Check sheet for the modelled part. Datum: model origin and axes. Units: mm. Round coordinates to 2 decimals unless told otherwise and drop trailing zeros. Order: outer loops, then holes, each group sorted by start corner. A loop starts at its lowest first (then second) coordinate and runs counter-clockwise, first axis right, second up. Notation, with made-up numbers: M 73,74 L 112,74 A23 ccw 112,82 Z; hole C 72,55.25 d7. An arc over 180 degrees is marked long. One line per item, written item: value. Start each with the question number.
(1) Cross-section at C-C, the plane y = 1.75. Enter the section's corners in (x, z).
(2) Cross-section at A-A, the plane x = -20. Enter the section's corners in (y, z).
(3) Cross-section at B-B, the plane z = 0.95. Enter the section's corners in (x, y).
(4) Release check for a two-part mould opening along X. For faces 1 (the face through (-20.737, 16.705, 0.986)), 2 (the face through (-22.5, 8, 1)), 3 (the face through (-17.5, 9, 1)), 4 (the face through (-20, 9, 2)) record: released by +X, released by -X, zero draft, split by the parting line, or undercut.
(5) Thickness scan on L1, parallel to Y at x = -20, z = 1.5; L2, parallel to X at y = 16, z = 0.9; L3, parallel to X at y = 0.5, z = 1.25. Record the ranges inside material, lowest first.
(6) Depth check by flat-ended pin: pin 1 Ø1.6 at (x, y) = (-20, 1.03) entering from -Z; pin 2 Ø2.5 at (x, y) = (-20, 16.03) entering from -Z. Enter the tip coordinate at first touch or a pass-through.
from build123d import *

# Parameters (mm, degrees)
SKETCH_1_R      = 1
EXTRUDE_2_DEPTH = 2
FILLET_1_R      = 0.3


with BuildPart() as part:
    # 草图1 → 凸台-拉伸2 (new body)
    with BuildSketch(Plane.XY):
        with BuildLine():
            Line((-22.5, 1.029411765), (-22.5, 16.029411765))
            ThreePointArc((-22.5, 16.029411765), (-20, 18.529411765), (-17.5, 16.029411765))
            Line((-17.5, 16.029411765), (-17.5, 1.029411765))
            ThreePointArc((-17.5, 1.029411765), (-20, -1.470588235), (-22.5, 1.029411765))
        make_face()
        with Locations((-20, 16.029411765)):
            Circle(SKETCH_1_R, mode=Mode.SUBTRACT)
        with Locations((-20, 1.029411765)):
            Circle(SKETCH_1_R, mode=Mode.SUBTRACT)
    extrude(amount=EXTRUDE_2_DEPTH)

    # 圆角1
    fillet_1_edges = [part.edges().sort_by_distance(p)[0] for p in [
        (-20, 18.529411765, 2),
        (-22.5, 8.529411765, 2),
        (-20, -1.470588235, 2),
        (-22.5, 8.529411765, 0),
        (-20, 18.529411765, 0),
        (-17.5, 8.529411765, 0),
        (-20, -1.470588235, 0),
        (-17.5, 8.529411765, 2),
    ]]
    fillet(fillet_1_edges, radius=FILLET_1_R)


solid = part.part
Values found:
1. outline: M -22.5,0.3 A0.3 ccw -22.2,0 L -20.69,0 L -20.69,2 L -22.2,2 A0.3 ccw -22.5,1.7 Z; M -19.31,0 L -17.8,0 A0.3 ccw -17.5,0.3 L -17.5,1.7 A0.3 ccw -17.8,2 L -19.31,2 Z
2. outline: M -1.47,0.3 A0.3 ccw -1.17,0 L 0.03,0 L 0.03,2 L -1.17,2 A0.3 ccw -1.47,1.7 Z; M 2.03,0 L 15.03,0 L 15.03,2 L 2.03,2 Z; M 17.03,0 L 18.23,0 A0.3 ccw 18.53,0.3 L 18.53,1.7 A0.3 ccw 18.23,2 L 17.03,2 Z
3. outline: M -22.5,1.03 A2.5 ccw -17.5,1.03 L -17.5,16.03 A2.5 ccw -22.5,16.03 Z; hole C -20,1.03 d2; hole C -20,16.03 d2
4. face 1: undercut
4. face 2: released by -X
4. face 3: released by +X
4. face 4: zero draft
5. L1: -1.47 to 0.03, 2.03 to 15.03, 17.03 to 18.53
5. L2: -22.5 to -21, -19 to -17.5
5. L3: -22.44 to -20.85, -19.15 to -17.56
6. pin 1: through
6. pin 2: z = 0
